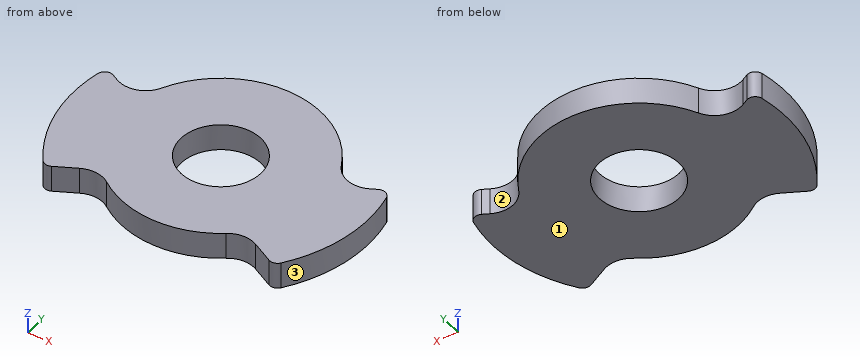
from build123d import *

# Parameters (mm, degrees)
F0_R     = 1.5
F1_DEPTH = 1


with BuildPart() as f1:
    # F0 (on Top) → F1 (new body)
    with BuildSketch(Plane.XY):
        with BuildLine():
            ThreePointArc((14.316125, 33.878389), (14.049917, 33.884634), (13.883606, 33.676676))
            ThreePointArc((13.883606, 33.676676), (13.877587, 31.360626), (14.82553, 29.247447))
            ThreePointArc((14.82553, 29.247447), (14.999791, 29.1328), (15.206672, 29.159473))
            Line((15.206672, 29.159473), (15.977662, 29.564092))
            ThreePointArc((15.977662, 29.564092), (16.517793, 29.675774), (17.034976, 29.484108))
            ThreePointArc((17.034976, 29.484108), (19.257285, 28.754678), (21.479594, 29.484108))
            ThreePointArc((21.479594, 29.484108), (21.996777, 29.675774), (22.536907, 29.564092))
            Line((22.536907, 29.564092), (23.307898, 29.159473))
            ThreePointArc((23.307898, 29.159473), (23.514778, 29.1328), (23.689039, 29.247447))
            ThreePointArc((23.689039, 29.247447), (24.636982, 31.360626), (24.630963, 33.676676))
            ThreePointArc((24.630963, 33.676676), (24.464653, 33.884634), (24.198444, 33.878389))
            Line((24.198444, 33.878389), (23.964436, 33.755581))
            ThreePointArc((23.964436, 33.755581), (23.194202, 33.68887), (22.60659, 34.191288))
            ThreePointArc((22.60659, 34.191288), (19.257285, 36.254678), (15.907979, 34.191288))
            ThreePointArc((15.907979, 34.191288), (15.320368, 33.68887), (14.550133, 33.755581))
            Line((14.550133, 33.755581), (14.316125, 33.878389))
        make_face()
        with Locations((19.257285, 32.504678)):
            Circle(F0_R, mode=Mode.SUBTRACT)
    extrude(amount=F1_DEPTH)


solid = f1.part
Source: CAD feature listing. Evaluate the final solid. Frame: model axes, mm. Face numbers are marked on the shaded views. Round coordinates to 2 decimals unless told otherwise and drop trailing zeros. Loops run counter-clockwise (first coordinate to the right, second up) from the corner with the lowest first, then second, coordinate; pieces in that order, holes last. Notation, with made-up numbers: M -40,20.25 L -5,20.25 A20 ccw -5,58.25 Z; hole C 24,86.5 d10. An arc over 180 degrees is marked long. Return JSON: item names as keys, results as strings. Group by question number.
1. Section query C-C on z = 0.8. Output: boundary loops of the cut face in (x, y), and give its area (3 significant figures).
2. Section query B-B on y = 31.25. Output: boundary loops of the cut face in (x, z).
3. Mould query, pull axis X, two halves, no side actions, for the marked faces 1, 2 and 3. Classes: released by +X, released by -X, zero draft, split by the parting line, or undercut.
4. Section query A-A on x = 18.75. Output: boundary loops of the cut face in (y, z), and give its area (3 significant figures).
5. Section query D-D on x = 16.75. Output: boundary loops of the cut face in (y, z).
6. Material intervals for line 1 along X through (y, z) = (32.5, 0.35); line 2 along X through (y, z) = (31.75, 0.1); line 3 along Y through (x, z) = (18.75, 0.75), sorted ascending. Write a range as from..to.
7. Pin query (flat end, axial travel): pin 1 (1.8 mm diameter, centred on x = 19.26, y = 32.5, fed in from -Z). Return the tip coordinate at first contact, or that it passes through.
Checks:
{
 "1": {"outline": "M 13.88,33.68 A5.5 ccw 14.83,29.25 A0.3 ccw 15.21,29.16 L 15.98,29.56 A1 cw 17.03,29.48 A3.75 ccw 21.48,29.48 A1 cw 22.54,29.56 L 23.31,29.16 A0.3 ccw 23.69,29.25 A5.5 ccw 24.63,33.68 A0.3 ccw 24.2,33.88 L 23.96,33.76 A1 cw 22.61,34.19 A3.75 ccw 15.91,34.19 A1 cw 14.55,33.76 L 14.32,33.88 A0.3 ccw Z; hole C 19.26,32.5 d3", "area": "53.4 mm²"},
 "2": {"outline": "M 13.9,0 L 18.44,0 L 18.44,1 L 13.9,1 Z; M 20.08,0 L 24.61,0 L 24.61,1 L 20.08,1 Z"},
 "3": {"face 1": "zero draft", "face 2": "undercut", "face 3": "released by +X"},
 "4": {"outline": "M 28.79,0 L 31.09,0 L 31.09,1 L 28.79,1 Z; M 33.92,0 L 36.22,0 L 36.22,1 L 33.92,1 Z", "area": "4.61 mm²"},
 "5": {"outline": "M 29.63,0 L 35.29,0 L 35.29,1 L 29.63,1 Z"},
 "6": {"line 1": "x = 13.76..17.76, 20.76..24.76", "line 2": "x = 13.81..17.96, 20.55..24.71", "line 3": "y = 28.79..31.09, 33.92..36.22"},
 "7": {"pin 1": "passes through"}
}
